Geometry check sheet. Reference: the model listing, model coordinates, mm. A direction names the side the tool comes from. Coordinates: 2 decimals unless noted, no trailing zeros. Write each loop counter-clockwise with the first axis right and the second up, starting at its lowest first coordinate (ties: lowest second). Pieces come first, ordered by that corner, then holes. Notation, with made-up numbers: (76, 29.25) - (112, 29.25) arc R33 cw to (112, 57.25) - close; hole circle Ø6 at (-21, 79). An arc over 180 degrees is marked (long way). Answer as a JSON object with one key per item and string values. Group by question number.
from build123d import *

# Parameters (mm, degrees)
SKETCH1_W           = 138
SKETCH1_H           = 47
BOSS_EXTRUDE1_DEPTH = 12.5
FILLET1_R           = 1.5
SKETCH2_W           = 8
SKETCH2_H           = 5
BOSS_EXTRUDE2_DEPTH = 5


with BuildPart() as part:
    # Sketch1 → Boss-Extrude1 (new, symmetric)
    with BuildSketch(Plane(origin=(0, 0, 0), x_dir=(1, 0, 0), z_dir=(0, 1, 0))):
        Rectangle(SKETCH1_W, SKETCH1_H)
    extrude(amount=BOSS_EXTRUDE1_DEPTH, both=True)

    # Fillet1
    fillet1_edges = [part.edges().sort_by_distance(p)[0] for p in [
        (-69, 12.5, 0),
        (0, 12.5, 23.5),
        (69, 12.5, 0),
        (0, -12.5, 23.5),
        (-69, -12.5, 0),
        (0, -12.5, -23.5),
        (69, -12.5, 0),
        (69, 0, 23.5),
        (-69, 0, 23.5),
        (-69, 0, -23.5),
        (69, 0, -23.5),
        (0, 12.5, -23.5),
    ]]
    fillet(fillet1_edges, radius=FILLET1_R)

    # Sketch2 → Boss-Extrude2 (add)
    with BuildSketch(Plane.ZY.offset(69)):
        with Locations((16, 6.5)):
            Rectangle(SKETCH2_W, SKETCH2_H)
    extrude(amount=BOSS_EXTRUDE2_DEPTH)


solid = part.part
(1) Section check B-B (z = 16). Record the cut outline in (x, y), and give its area (3 significant figures).
(2) Material ranges on L1, parallel to X at y = -4.5, z = -7; L2, parallel to X at y = 11.5, z = -5.5, recorded low to high. Write a range as [from, to].
(3) Gauge pin test, flat ends, axial feed: pin 1 (2.5 mm diameter, centred on x = -71.5, y = 7, fed in from -Z); pin 2 (4 mm diameter, centred on x = -70.5, y = 6.5, fed in from +Z); pin 3 (11 mm diameter, centred on y = -5.5, z = -1, fed in from -X). Record the tip position at first contact, or that the pin passes through.
(4) Section check A-A (y = 2.75). Record the cut outline in (x, z), and give its area (3 significant figures).
(5) Set-up check for faces 1 (the face through (-71, 9, 16)), 2 (the face through (-71, 4, 16)), 3 (the face through (-71, 6, 20)), 4 (the face through (-71, 6, 12)): record each of +Z, -Z, +X, -X, +Y, -Y from which the full face is reachable in a straight line by a thin tool's end or side.
(6) Section check C-C (z = -16.5). Record the cut outline in (x, y).
Conclusion:
{
 "1": {"outline": "(-74, 4) - (-69, 4) - (-69, -11) arc R1.5 ccw to (-67.5, -12.5) - (67.5, -12.5) arc R1.5 ccw to (69, -11) - (69, 11) arc R1.5 ccw to (67.5, 12.5) - (-67.5, 12.5) arc R1.5 ccw to (-69, 11) - (-69, 9) - (-74, 9) - close", "area": "3,470 mm^2"},
 "2": {"L1": "x = [-69, 69]", "L2": "x = [-68.91, 68.91]"},
 "3": {"pin 1": "stops at z = 12", "pin 2": "stops at z = 23.12", "pin 3": "stops at x = -69"},
 "4": {"outline": "(-69, -22) arc R1.5 ccw to (-67.5, -23.5) - (67.5, -23.5) arc R1.5 ccw to (69, -22) - (69, 22) arc R1.5 ccw to (67.5, 23.5) - (-67.5, 23.5) arc R1.5 ccw to (-69, 22) - close", "area": "6,480 mm^2"},
 "5": {"face 1": "+Z, -Z, -X, +Y", "face 2": "+Z, -Z, -X, -Y", "face 3": "+Z, -X, +Y, -Y", "face 4": "-Z, -X, +Y, -Y"},
 "6": {"outline": "(-69, -11) arc R1.5 ccw to (-67.5, -12.5) - (67.5, -12.5) arc R1.5 ccw to (69, -11) - (69, 11) arc R1.5 ccw to (67.5, 12.5) - (-67.5, 12.5) arc R1.5 ccw to (-69, 11) - close"}
}
